Source: CAD feature listing. Evaluate the final solid. Frame: model axes, mm. A direction names the side the tool comes from. Round coordinates to 2 decimals unless told otherwise and drop trailing zeros. Order: outer loops, then holes, each group sorted by start corner. A loop starts at its lowest first (then second) coordinate and runs counter-clockwise, first axis right, second up. Notation, with made-up numbers: M 76,-33 L 86,-33 A26 cw 86,-10 Z; hole C 33,22 d8. An arc over 180 degrees is marked long. Use one line per item in the form item = value. Start each with the question number.
Q1. Section D-D (z = 15.5). Return the cut outline in (x, y).
Q2. Reachability of faces 4 (the cylindrical face through (-41, 5, 0)), 5 (the flat face through (22, 43, 0)), 6 (the flat face through (0, 13, 0)), 7 (the cylindrical face through (57.5, 7.9, 0.1)) from +Z, -Z, +X, -X, +Y, -Y: full face, straight path, thin tool, end or side. Return the list, or none.
Q3. Material intervals for probe 1 along Z at (x, y) = (-31, 7.75); probe 2 along X at (y, z) = (27.5, 4); probe 3 along X at (y, z) = (5.5, -4.5), sorted ascending.
Q4. Pull-direction query (Z, two-part tool) for faces 1 (the cylindrical face through (-43, 34, 0)), 2 (the flat face through (-64, 8, 2.5)), 3 (the flat face through (-1, 0, 0)); classes: pulls with the +Z half, pulls with the -Z half, needs draft (parallel to the pull), parting line crosses it, or undercut.
Q5. Contact query for flat-ended pins moving along their axis: pin 1 (0.9 mm diameter, centred on x = 22.5, z = 8.5, fed in from +Y); pin 2 (1 mm diameter, centred on y = 1.5, z = -2.5, fed in from -X); pin 3 (7 mm diameter, centred on x = 0, z = 0, fed in from +Y). Output: stop coordinate, or through.
Q6. Section C-C (x = -51.5). Return the cut outline in (y, z).
Q7. Section A-A (x = -31). Return the cut outline in (y, z).
from build123d import *

# Parameters (mm, degrees)
BOSS_EXTRUDE1_DEPTH = 19
CUT_EXTRUDE2_DEPTH  = 2
BOSS_EXTRUDE2_DEPTH = 41
CUT_EXTRUDE3_DEPTH  = 62
SKETCH6_R           = 5.25
CUT_EXTRUDE4_DEPTH  = 72
SKETCH7_R           = 10
CUT_EXTRUDE5_DEPTH  = 9
SKETCH8_R           = 6
CUT_EXTRUDE6_DEPTH  = 42


with BuildPart() as part:
    # Sketch2 → Boss-Extrude1 (new, symmetric)
    with BuildSketch(Plane.XY):
        Polygon((-84, 0), (0, 0), (84, 0), (80, 14), (-80, 14), align=None)
    extrude(amount=BOSS_EXTRUDE1_DEPTH, both=True)

    # Sketch3 → Cut-Extrude2 (cut)
    with BuildSketch(Plane.XZ):
        Polygon((-76, 11), (-76, 0), (-76, -11), (-8, -11), (-8, 11), align=None)
        Polygon((76, 0), (76, -11), (8, -11), (8, 11), (76, 11), align=None)
    extrude(amount=-CUT_EXTRUDE2_DEPTH, mode=Mode.SUBTRACT)

    # Sketch4 → Boss-Extrude2 (add)
    with BuildSketch(Plane(origin=(0, 14, 0), x_dir=(1, 0, 0), z_dir=(0, 1, 0))):
        with BuildLine():
            Line((-38.574603044, 19), (38.574603044, 19))
            ThreePointArc((38.574603044, 19), (43, 0), (38.574603044, -19))
            Line((38.574603044, -19), (-38.574603044, -19))
            ThreePointArc((-38.574603044, -19), (-43, 0), (-38.574603044, 19))
        make_face()
    extrude(amount=BOSS_EXTRUDE2_DEPTH)

    # Sketch5 → Cut-Extrude3 (cut)
    with BuildSketch(Plane.XY.offset(19)):
        with BuildLine():
            Line((20.674705774, 39.999892181), (20.674705774, 43))
            Line((20.674705774, 43), (23.674705774, 43))
            Line((23.674705774, 43), (23.674705774, 55))
            Line((23.674705774, 55), (-20.325294226, 55))
            Line((-20.325294226, 55), (-20.325294226, 43))
            Line((-20.325294226, 43), (-17.325294226, 43))
            Line((-17.325294226, 43), (-17.325294226, 39.999892181))
            ThreePointArc((-17.325294226, 39.999892181), (1.674705774, 20.999892181), (20.674705774, 39.999892181))
        make_face()
    extrude(amount=-CUT_EXTRUDE3_DEPTH, mode=Mode.SUBTRACT)

    # Sketch6 → Cut-Extrude4 (cut)
    with BuildSketch(Plane.XZ):
        with Locations((-31, 0)):
            Circle(SKETCH6_R)
        with Locations(Location((31, 0, 0), (0, 0, 90))):
            Circle(SKETCH6_R)
        with BuildLine():
            Line((68, 2.5), (60, 2.5))
            ThreePointArc((60, 2.5), (57.5, 0), (60, -2.5))
            Line((60, -2.5), (68, -2.5))
            ThreePointArc((68, -2.5), (70.5, 0), (68, 2.5))
        make_face()
        with BuildLine():
            Line((-68, 2.5), (-60, 2.5))
            ThreePointArc((-60, 2.5), (-57.5, 0), (-60, -2.5))
            Line((-60, -2.5), (-68, -2.5))
            ThreePointArc((-68, -2.5), (-70.5, 0), (-68, 2.5))
        make_face()
    extrude(amount=-CUT_EXTRUDE4_DEPTH, mode=Mode.SUBTRACT)

    # Sketch7 → Cut-Extrude5 (cut)
    with BuildSketch(Plane.XZ):
        with Locations((-31, 0)):
            Circle(SKETCH7_R)
        with Locations((31, 0)):
            Circle(SKETCH7_R)
    extrude(amount=-CUT_EXTRUDE5_DEPTH, mode=Mode.SUBTRACT)

    # Sketch8 → Cut-Extrude6 (cut)
    with BuildSketch(Plane(origin=(0, 55, 0), x_dir=(1, 0, 0), z_dir=(0, 1, 0))):
        with Locations(Location((0, 0, 0), (0, 0, 270))):
            Circle(SKETCH8_R)
    extrude(amount=-CUT_EXTRUDE6_DEPTH, mode=Mode.SUBTRACT)


solid = part.part
Results list:
q1.outline = M -84,0 L 84,0 L 80,14 L 40.11,14 L 40.11,55 L 23.67,55 L 23.67,43 L 20.67,43 L 20.67,40 A19 cw -17.33,40 L -17.33,43 L -20.33,43 L -20.33,55 L -40.11,55 L -40.11,14 L -80,14 Z
q2.face_4 = -Y
q2.face_5 = +Z, -Z, +Y
q2.face_6 = +Y
q2.face_7 = +Y, -Y
q3.probe_1 = -19 to -10, 10 to 19
q3.probe_2 = -42.81 to -34.4, -27.6 to -12.63, 15.98 to 27.6, 34.4 to 42.81
q3.probe_3 = -82.43 to -39.93, -22.07 to 22.07, 39.93 to 82.43
q4.face_1 = parting line crosses it
q4.face_2 = undercut
q4.face_3 = needs draft
q5.pin_1 = 43
q5.pin_2 = -83.71
q5.pin_3 = 13
q6.outline = M 0,-19 L 14,-19 L 14,19 L 0,19 L 0,11 L 2,11 L 2,-11 L 0,-11 Z
q7.outline = M 0,-19 L 55,-19 L 55,-5.25 L 9,-5.25 L 9,-10 L 2,-10 L 2,-11 L 0,-11 Z; M 0,11 L 2,11 L 2,10 L 9,10 L 9,5.25 L 55,5.25 L 55,19 L 0,19 Z
